Geometry: final body of the model. Coordinates: model frame, mm. A direction names the side the tool comes from. Give positions to 0.01 mm unless a question says otherwise; leave off trailing zeros. Write each loop counter-clockwise with the first axis right and the second up, starting at its lowest first coordinate (ties: lowest second). Pieces come first, ordered by that corner, then holes.
Q1. Mould query, pull axis Z, two halves, no side actions, for faces 1 (the flat face through (-1, 0, 16)), 2 (the cylindrical face through (-58.23, 11.83, -53.39)), 3 (the cylindrical face through (-22.993, 20.838, -51.691)). Classes: +Z half, -Z half, draft (parallel to the pull), parting line (faces both ways), or undercut.
Q2. Section A-A (x = 0). Return the cut outline in (y, z), plus the area to 3 significant figures.
Q3. Line query: line 1 (Z direction, x = -32, y = 20.5); line 2 (X direction, y = 20.5, z = -48); line 3 (Z direction, x = 32, y = 19.5). Output: solid intervals per line, ascending.
Q4. Pin query (flat end, axial travel): pin 1 Ø2 at (y, z) = (3.5, 40) entering from -X; pin 2 Ø10 at (x, z) = (33.5, -57) entering from +Y; pin 3 Ø10 at (y, z) = (10.5, -27) entering from -X. Return the tip coordinate at first contact, or that it passes through.
Q5. Section B-B (y = 3.25). Return the cut outline in (x, z).
Q6. Reachability of faces 4 (the cylindrical face through (29.12, 7.15, -49.88)), 5 (the flat face through (32, 14.5, 62)) from +Z, -Z, +X, -X, +Y, -Y: full face, straight path, thin tool, end or side. Return the list, or none.
from build123d import *

# Parameters (mm, degrees)
SKETCH1_R                                           = 79
SKETCH1_R_2                                         = 12
BOSS_EXTRUDE3_DEPTH                                 = 27
CBORE_FOR_00_BINDING_HEAD_MACHINE_SCREW_D           = 12.499999892
CBORE_FOR_00_BINDING_HEAD_MACHINE_SCREW_CBORE_D     = 19.500000116
CBORE_FOR_00_BINDING_HEAD_MACHINE_SCREW_CBORE_DEPTH = 12.499999892
F_97_0_0059_DIAMETER_HOLE1_D                        = 13.99999994
F_97_0_0059_DIAMETER_HOLE1_DEPTH                    = 17
F_97_0_0059_DIAMETER_HOLE1_TIP                      = 4.206024315
SKETCH8_R                                           = 33
SKETCH8_R_2                                         = 22
CUT_EXTRUDE1_DEPTH                                  = 6
CHAMFER1_SIZE                                       = 3


with BuildPart() as part:
    # Sketch1 → Boss-Extrude3 (new body)
    with BuildSketch(Plane(origin=(0, 0, 0), x_dir=(1, 0, 0), z_dir=(0, 1, 0))):
        Circle(SKETCH1_R)
        Circle(SKETCH1_R_2, mode=Mode.SUBTRACT)
    extrude(amount=BOSS_EXTRUDE3_DEPTH)

    # CBORE for #00 Binding Head Machine Screw1 (through all)
    with Locations(Plane(origin=(0, 27, 0), x_dir=(1, 0, 0), z_dir=(0, 1, 0))):
        with Locations((32, 55.425625842), (64, 0), (32, -55.425625842), (-32, -55.425625842), (-64, 0), (-32, 55.425625842), (0, 0)):
            CounterBoreHole(CBORE_FOR_00_BINDING_HEAD_MACHINE_SCREW_D / 2, CBORE_FOR_00_BINDING_HEAD_MACHINE_SCREW_CBORE_D / 2, CBORE_FOR_00_BINDING_HEAD_MACHINE_SCREW_CBORE_DEPTH)

    # #97 (0.0059) Diameter Hole1
    with Locations(Plane(origin=(0, 27, 0), x_dir=(1, 0, 0), z_dir=(0, 1, 0))):
        with Locations((34, 0)):
            Hole(F_97_0_0059_DIAMETER_HOLE1_D / 2, depth=F_97_0_0059_DIAMETER_HOLE1_DEPTH)
            with Locations((0, 0, -(F_97_0_0059_DIAMETER_HOLE1_DEPTH + F_97_0_0059_DIAMETER_HOLE1_TIP / 2))):  # 118° drill point
                Cone(0, F_97_0_0059_DIAMETER_HOLE1_D / 2, F_97_0_0059_DIAMETER_HOLE1_TIP, mode=Mode.SUBTRACT)

    # Sketch8 → Cut-Extrude1 (cut)
    with BuildSketch(Plane(origin=(0, 27, 0), x_dir=(1, 0, 0), z_dir=(0, 1, 0))):
        Circle(SKETCH8_R)
        Circle(SKETCH8_R_2, mode=Mode.SUBTRACT)
    extrude(amount=-CUT_EXTRUDE1_DEPTH, mode=Mode.SUBTRACT)

    # Chamfer1
    chamfer1_edges = [part.edges().sort_by_distance(p)[0] for p in [
        (-79, 27, 0),
    ]]
    chamfer(chamfer1_edges, length=CHAMFER1_SIZE)


solid = part.part
Computed:
1. face 1: draft
1. face 2: parting line
1. face 3: undercut
2. outline: (0, -79) - (24, -79) - (27, -76) - (27, -33) - (21, -33) - (21, -22) - (27, -22) - (27, -12) - (0, -12) - close; (0, 12) - (27, 12) - (27, 22) - (21, 22) - (21, 33) - (27, 33) - (27, 76) - (24, 79) - (0, 79) - close
2. area: 3,480 mm2
3. line 1: z = -72.23 to -65.18, -45.68 to 45.68, 65.18 to 72.23
3. line 2: x = -62.75 to -38.32, -25.68 to 25.68, 38.32 to 62.75
3. line 3: z = -72.23 to -65.18, -45.68 to -6.71, 6.71 to 45.68, 65.18 to 72.23
4. pin 1: stops at x = -68.7
4. pin 2: stops at y = 14.5
4. pin 3: stops at x = -75.87
5. outline: circle Ø158 at (0, 0); hole circle Ø12.5 at (-64, 0); hole circle Ø12.5 at (-32, -55.43); hole circle Ø12.5 at (-32, 55.43); hole circle Ø24 at (0, 0); hole circle Ø12.5 at (32, -55.43); hole circle Ø12.5 at (32, 55.43); hole circle Ø12.5 at (64, 0)
6. face 4: +Y, -Y
6. face 5: +Y
